CAD build for the part. Positions are in the model's coordinates, mm. A direction names the side the tool comes from. Round coordinates to 2 decimals unless told otherwise and drop trailing zeros. Loops run counter-clockwise (first coordinate to the right, second up) from the corner with the lowest first, then second, coordinate; pieces in that order, holes last. Notation, with made-up numbers: M -21.5,1.5 L 25.5,1.5 A19 cw 25.5,20.5 Z; hole C -13,-10 d2. An arc over 180 degrees is marked long. Use one line per item in the form item = value.
from build123d import *

# Parameters (mm, degrees)
BOSS_EXTRUDE1_DEPTH                  = 5
BOSS_EXTRUDE1_DEPTH_BACK             = 5
SKETCH1_W                            = 100
SKETCH1_H                            = 100
SKETCH2_R                            = 8.75
SKETCH2_R_2                          = 3.25
CUT_EXTRUDE1_DEPTH                   = 12.7
TAP_DRILL_FOR_M5X0_8_TAP1_AT_2_COUNT = 2
TAP_DRILL_FOR_M5X0_8_TAP1_AT_2_PITCH = 70
SKETCH11_R                           = 37.5
CUT_EXTRUDE2_DEPTH                   = 3
CHAMFER1_SIZE                        = 0.5
SKETCH12_R                           = 1.75
CUT_EXTRUDE3_DEPTH                   = 72.414284285
SKETCH13_R                           = 2.25
CUT_EXTRUDE4_DEPTH                   = 10
SKETCH14_R                           = 1.5
CUT_EXTRUDE5_DEPTH                   = 10


with BuildPart() as part:
    # Sketch1 → Boss-Extrude1 (new, two sides: drawn at the far end of the back side and taken through both)
    with BuildSketch(Plane(origin=(0, 0, 0), x_dir=(1, 0, 0), z_dir=(0, 1, 0)).offset(-BOSS_EXTRUDE1_DEPTH_BACK)):
        Rectangle(SKETCH1_W, SKETCH1_H)
    extrude(amount=BOSS_EXTRUDE1_DEPTH + BOSS_EXTRUDE1_DEPTH_BACK)

    # Sketch2 → Cut-Extrude1 (cut)
    with BuildSketch(Plane(origin=(0, 5, 0), x_dir=(1, 0, 0), z_dir=(0, 1, 0))):
        with Locations(Location((0, 0, 0), (0, 0, 270))):
            Circle(SKETCH2_R)
        with Locations(Location((-34.798492469, 34.798492469, 0), (0, 0, 270))):
            Circle(SKETCH2_R_2)
        with Locations(Location((34.798492469, 34.798492469, 0), (0, 0, 270))):
            Circle(SKETCH2_R_2)
        with Locations(Location((34.798492469, -34.798492469, 0), (0, 0, 270))):
            Circle(SKETCH2_R_2)
        with Locations(Location((-34.798492469, -34.798492469, 0), (0, 0, 270))):
            Circle(SKETCH2_R_2)
    extrude(amount=-CUT_EXTRUDE1_DEPTH, mode=Mode.SUBTRACT)

    # Sketch10 → Tap Drill for M5x0.8 Tap1 (revolve, cut)
    with BuildSketch(Plane(origin=(-50, 0, -35), x_dir=(0, 0, 1), z_dir=(0, 1, 0))):
        Polygon((0, 0), (0, 11.2618073), (2.1, 10), (2.1, 0), align=None)
    tap_drill_for_m5x0_8_tap1 = revolve(axis=Axis((-56.35, 0, -35), (1, 0, 0)), mode=Mode.SUBTRACT)

    # Tap Drill for M5x0.8 Tap1 at 2: Tap Drill for M5x0.8 Tap1 ×2
    with Locations(*[(0, 0, i * TAP_DRILL_FOR_M5X0_8_TAP1_AT_2_PITCH) for i in range(1, TAP_DRILL_FOR_M5X0_8_TAP1_AT_2_COUNT)]):
        add(tap_drill_for_m5x0_8_tap1, mode=Mode.SUBTRACT)

    # Sketch11 → Cut-Extrude2 (cut)
    with BuildSketch(Plane.XZ.offset(5)):
        with Locations(Location((0, 0, 0), (0, 0, 270))):
            Circle(SKETCH11_R)
    extrude(amount=-CUT_EXTRUDE2_DEPTH, mode=Mode.SUBTRACT)

    # Chamfer1
    chamfer1_edges = [part.edges().sort_by_distance(p)[0] for p in [
        (-50, 0, -50),
        (50, 0, -50),
        (50, 0, 50),
        (-50, 0, 50),
    ]]
    chamfer(chamfer1_edges, length=CHAMFER1_SIZE)

    # Mirror1: Tap Drill for M5x0.8 Tap1 across plane
    add(tap_drill_for_m5x0_8_tap1.mirror(Plane.ZY), mode=Mode.SUBTRACT)

    # Mirror1 copy 1 sketch → Mirror1 copy 1 (revolve, cut)
    with BuildSketch(Plane(origin=(50, 0, 35), x_dir=(0, 0, 1), z_dir=(0, 1, 0))):
        Polygon((0, 0), (0, -11.2618073), (2.1, -10), (2.1, 0), align=None)
    revolve(axis=Axis((56.35, 0, 35), (1, 0, 0)), mode=Mode.SUBTRACT)

    # Sketch12 → Cut-Extrude3 (cut, through all)
    with BuildSketch(Plane(origin=(0, 5, 0), x_dir=(1, 0, 0), z_dir=(0, 1, 0))):
        with Locations(Location((7.75, 20.423393759, 0), (0, 0, 270))):
            Circle(SKETCH12_R)
        with Locations(Location((-7.75, 20.423393759, 0), (0, 0, 270))):
            Circle(SKETCH12_R)
        with Locations(Location((15.5, 7, 0), (0, 0, 90))):
            Circle(SKETCH12_R)
        with Locations((7.75, -6.423393759)):
            Circle(SKETCH12_R)
        with Locations((-7.75, -6.423393759)):
            Circle(SKETCH12_R)
        with Locations(Location((-15.5, 7, 0), (0, 0, 270))):
            Circle(SKETCH12_R)
    extrude(amount=-CUT_EXTRUDE3_DEPTH, mode=Mode.SUBTRACT)

    # Sketch13 → Cut-Extrude4 (cut)
    with BuildSketch(Plane(origin=(0, 5, 0), x_dir=(1, 0, 0), z_dir=(0, 1, 0))):
        with Locations(Location((-15.5, -15.5, 0), (0, 0, 270))):
            Circle(SKETCH13_R)
        with Locations(Location((-15.5, 15.5, 0), (0, 0, 270))):
            Circle(SKETCH13_R)
        with Locations(Location((15.5, 15.5, 0), (0, 0, 270))):
            Circle(SKETCH13_R)
        with Locations(Location((15.5, -15.5, 0), (0, 0, 270))):
            Circle(SKETCH13_R)
    extrude(amount=-CUT_EXTRUDE4_DEPTH, mode=Mode.SUBTRACT)

    # Sketch14 → Cut-Extrude5 (cut)
    with BuildSketch(Plane(origin=(0, 5, 0), x_dir=(1, 0, 0), z_dir=(0, 1, 0))):
        with Locations(Location((0, 11, 0), (0, 0, 270))):
            Circle(SKETCH14_R)
        with Locations(Location((-11, 0, 0), (0, 0, 270))):
            Circle(SKETCH14_R)
        with Locations(Location((0, -11, 0), (0, 0, 270))):
            Circle(SKETCH14_R)
        with Locations(Location((11, 0, 0), (0, 0, 270))):
            Circle(SKETCH14_R)
    extrude(amount=-CUT_EXTRUDE5_DEPTH, mode=Mode.SUBTRACT)


solid = part.part
1. Cut at D-D on y = 3.75. State how many separate pieces and enclosed holes the cut face has, and give its area (3 significant figures).
Completed:
separate_pieces = 1
enclosed_holes = 17
area = 9,480 mm2
2. Cut at A-A on z = 0. Write the cut outline in (x, y), and give its area (4 significant figures).
Completed:
outline = M -50,-5 L -37.5,-5 L -37.5,-2 L -12.5,-2 L -12.5,5 L -50,5 Z; M -9.5,-2 L -8.75,-2 L -8.75,5 L -9.5,5 Z; M 8.75,-2 L 9.5,-2 L 9.5,5 L 8.75,5 Z; M 12.5,-2 L 37.5,-2 L 37.5,-5 L 50,-5 L 50,5 L 12.5,5 Z
area = 610.5 mm2
3. Cut at B-B on x = -11. Write the cut outline in (y, z).
Completed:
outline = M -5,-50 L 5,-50 L 5,-1.5 L -2,-1.5 L -2,-35.85 L -5,-35.85 Z; M -5,35.85 L -2,35.85 L -2,1.5 L 5,1.5 L 5,50 L -5,50 Z
4. Drop a flat-ended pin along its axis: P1, Ø4.5, axis at x = 7.75, z = -20.42, coming from the -Y side. Give the stop position or say it passes through.
Completed:
P1 = -2
5. Tool access for faces 5 (the face through (-0.09, 1.55, 8.75)), 6 (the face through (-12, 5, -12)), 7 (the face through (-45.07, -0.09, -37.1)), 8 (the face through (45.07, -0.09, 32.9)): list every direction of +Z, -Z, +X, -X, +Y, -Y with a clear straight run to the whole face (end or side of a thin tool).
Completed:
face_5 = +Y, -Y
face_6 = +Z, -Z, +X, -X, +Y
face_7 = -X
face_8 = +X
6. Pull direction X, two halves, no side cores. Call faces 1 (the face through (-37.97, 0.07, 34.09)), 2 (the face through (-23, -5, -34)), 3 (the face through (-38.957, -0.016, 34.636)), 4 (the face through (50, 0, 1)): +X half, -X half, draft (parallel to the pull), parting line (faces both ways), or undercut.
Completed:
face_1 = undercut
face_2 = draft
face_3 = -X half
face_4 = +X half
7. Cut at C-C on z = 15. Write the cut outline in (x, y).
Completed:
outline = M -50,-5 L -34.37,-5 L -34.37,-2 L -17.69,-2 L -17.69,5 L -50,5 Z; M -13.31,-2 L 13.31,-2 L 13.31,5 L -13.31,5 Z; M 17.69,-2 L 34.37,-2 L 34.37,-5 L 50,-5 L 50,5 L 17.69,5 Z
8. Probe line 1 along X through (y, z) = (2.75, 15.5); line 2 along Z through (x, y) = (44.5, 0); line 3 along X through (y, z) = (-1, 1). List the from-to ranges inside material, lowest first. Write a range as from..to.
Completed:
line_1 = -50..-17.75, -13.25..13.25, 17.75..50
line_2 = -50..-37.1, -32.9..32.9, 37.1..50
line_3 = -50..-12.12, -9.88..-8.69, 8.69..9.88, 12.12..50
